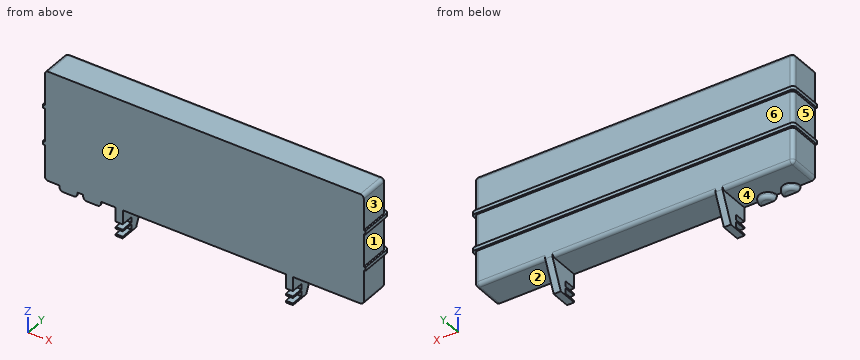
Autodesk Fusion 360 part; units mm, degrees
sketch "Sketch1" plane through (0, 0, 0) normal (0, 1, 0) x (1, 0, 0)
  line L0 (0, 0) -> (90, 0)
  line L1 (90, 0) -> (90, 31)
  line L2 (90, 31) -> (0, 31)
  line L3 (0, 31) -> (0, 0)
  line L4 (-3, 20.67) -> (93, 20.67) construction
  line L5 (-3, 10.33) -> (93, 10.33) construction
  line L6 (0, 21.17) -> (90, 21.17)
  line L7 (0, 20.17) -> (90, 20.17)
  line L8 (0, 9.83) -> (90, 9.83)
  line L9 (0, 10.83) -> (90, 10.83)
  line L10 (90, 20.17) -> (90.5, 20.17)
  line L11 (90.5, 20.17) -> (90.5, 21.17)
  line L12 (90.5, 21.17) -> (90, 21.17)
  line L13 (90, 21.17) -> (90, 20.17)
  line L14 (90, 10.83) -> (90.5, 10.83)
  line L15 (90.5, 10.83) -> (90.5, 9.83)
  line L16 (90.5, 9.83) -> (90, 9.83)
  line L17 (90, 9.83) -> (90, 10.83)
  line L18 (0, 21.17) -> (-0.5, 21.17)
  line L19 (-0.5, 21.17) -> (-0.5, 20.17)
  line L20 (-0.5, 20.17) -> (0, 20.17)
  line L21 (0, 20.17) -> (0, 21.17)
  line L22 (0, 9.83) -> (-0.5, 9.83)
  line L23 (-0.5, 9.83) -> (-0.5, 10.83)
  line L24 (-0.5, 10.83) -> (0, 10.83)
  line L25 (0, 10.83) -> (0, 9.83)
  line L26 (70, 39) -> (68, 39)
  line L27 (68, 39) -> (68, 38.5)
  line L28 (68, 38.5) -> (70, 38.5)
  line L29 (70, 38.5) -> (70, 39)
  line L30 (68, 37) -> (70, 37)
  line L31 (70, 37) -> (70, 36.5)
  line L32 (70, 36.5) -> (68, 36.5)
  line L33 (68, 36.5) -> (68, 37)
  line L34 (20, 37) -> (22, 37)
  line L35 (22, 37) -> (22, 36.5)
  line L36 (22, 36.5) -> (20, 36.5)
  line L37 (20, 36.5) -> (20, 37)
  line L38 (20, 38.5) -> (22, 38.5)
  line L39 (22, 38.5) -> (22, 39)
  line L40 (22, 39) -> (20, 39)
  line L41 (20, 39) -> (20, 38.5)
  dimension "d1" = 90
  dimension "d2" = 31
  dimension "d3" = 10.33
  dimension "d4" = 10.33
  dimension "d5" = 0.5
  dimension "d6" = 0.5
  dimension "d7" = 0.5
  dimension "d8" = 0.5
  dimension "d9" = 0.5
  dimension "d10" = 0.5
  dimension "d11" = 0.5
  dimension "d12" = 0.5
  dimension "d84" = 0.5
  dimension "d86" = 8
  dimension "d88" = 2
  dimension "d89" = 0.5
  dimension "d90" = 0.5
  dimension "d91" = 20
  dimension "d92" = 20
  dimension "d93" = 20
  dimension "d94" = 0.5
  dimension "d95" = 8
  dimension "d96" = 6
  dimension "d97" = 6
extrude "Extrude1" add sketch "Sketch1" along normal blind 9 contours L1 L2 L3 L6 makes body 1
extrude "Extrude2" add sketch "Sketch1" along normal blind 9 separate body contours L1 L3 L7 L9 makes body 2
extrude "Extrude3" add sketch "Sketch1" along normal blind 9 separate body contours L0 L1 L3 L8 makes body 3
extrude "Extrude4" add sketch "Sketch1" along normal blind 9.5 contours L1 L3 L6 L7 L13 L21 bodies 1 2
extrude "Extrude5" add sketch "Sketch1" along normal blind 9.5 contours L1 L3 L8 L9 L17 L25 bodies 1 3
extrude "Extrude6" add sketch "Sketch1" along normal blind 9.5 contours L1 L10 L11 L12 L13 bodies 1
extrude "Extrude7" add sketch "Sketch1" along normal blind 9.5 contours L1 L14 L15 L16 L17 bodies 1
extrude "Extrude8" add sketch "Sketch1" along normal blind 9.5 contours L3 L18 L19 L20 L21 bodies 1
extrude "Extrude9" add sketch "Sketch1" along normal blind 9.5 contours L3 L22 L23 L24 L25 bodies 1
sketch "Sketch2" plane through (0, 0, 0) normal (1, 0, 0) x (0, 0, -1)
  line L0 (39, 0) -> (31, 0)
  line L1 (31, 0) -> (31, 5.5)
  line L2 (31, 5.5) -> (39, 5.5)
  line L3 (39, 5.5) -> (39, 0)
  line L4 (31, 9) -> (39, 5.5)
  line L5 (31, 9) -> (31, 5.5)
  line L6 (39, 0) -> (35, 0)
  line L7 (35, 0) -> (35, 3.5)
  line L8 (35, 3.5) -> (39, 3.5)
  line L9 (39, 3.5) -> (39, 0)
  point P0 (31, 0)
  dimension "d33" = 8
  dimension "d34" = 8
  dimension "d35" = 5.5
  dimension "d36" = 3.5
  dimension "d37" = 4
extrude "Extrude10" add sketch "Sketch2" along normal blind 2 from surface at 68 contours L0 L1 L2 L3 L7 L8 | L2 L4 L5 bodies 1
extrude "Extrude11" add sketch "Sketch2" along normal blind 2 from surface at 20 contours L0 L1 L2 L3 L7 L8 | L2 L4 L5 bodies 1
fillet "Fillet1" radius 1 1 edges at (90, 9, -4.915) on bodies 1
fillet "Fillet2" radius 1 1 edges at (90, 9, -15.5) on bodies 1
fillet "Fillet3" radius 1 1 edges at (90, 9, -26.085) on bodies 1
fillet "Fillet4" radius 1 3 edges at (90, 4, -31) (89.7071, 8.7071, -31) (79.5, 9, -31) on bodies 1
fillet "Fillet5" radius 1 3 edges at (90, 4, 0) (89.7071, 8.7071, 0) (44.5, 9, 0) on bodies 1
fillet "Fillet6" radius 1 3 edges at (0, 4, 0) (0, 8.7071, -0.2929) (0, 9, -5.415) on bodies 1
fillet "Fillet7" radius 1 1 edges at (0, 9, -15.5) on bodies 1
fillet "Fillet8" radius 1 1 edges at (0, 9, -26.085) on bodies 1
fillet "Fillet9" radius 1 3 edges at (0, 4, -31) (0.2929, 8.7071, -31) (10.5, 9, -31) on bodies 1
fillet "Fillet10" radius 1 1 edges at (45, 9, -31) on bodies 1
sketch "Sketch3" plane through (0, 0, -31) normal (0, 0, -1) x (-1, 0, 0)
  line L0 (-1, 8) -> (-20, 8)
  line L1 (-20, 8) -> (-20, 0)
  line L2 (-20, 0) -> (-1, 0)
  line L3 (-1, 0) -> (-1, 8)
  line L4 (-6.666, -3) -> (-6.666, 13) construction
  line L5 (-13.333, -2) -> (-13.333, 13) construction
  circle A0 centre (-6.666, 0) radius 2.5
  circle A1 centre (-13.333, 0) radius 2.5
  dimension "d64" = 6.667
  dimension "d65" = 6.667
  dimension "d66" = 5
  dimension "d67" = 5
extrude "Extrude12" add sketch "Sketch3" along normal blind 1.5 contours L2 A0 picked at (-6.0551, 0.5668) bodies 1
extrude "Extrude13" add sketch "Sketch3" along normal blind 1.5 contours L2 A1 picked at (-12.6445, 0.4694) bodies 1
fillet "Fillet11" radius 1 1 edges at (6.666, 2.5, -32.5) on bodies 1
fillet "Fillet12" radius 1 1 edges at (13.333, 2.5, -32.5) on bodies 1
fillet "Fillet13" radius 1 1 edges at (90.5, 9.5, -20.67) on bodies 1
fillet "Fillet14" radius 1 1 edges at (90.5, 9.5, -10.33) on bodies 1
fillet "Fillet15" radius 1 1 edges at (-0.5, 9.5, -20.67) on bodies 1
fillet "Fillet16" radius 1 1 edges at (-0.5, 9.5, -10.33) on bodies 1
extrude "Extrude14" add sketch "Sketch1" along normal blind 3.5 contours L26 L27 L28 L29 | L30 L31 L32 L33 bodies 1
extrude "Extrude15" add sketch "Sketch1" along normal blind 3.5 contours L34 L35 L36 L37 | L38 L39 L40 L41 bodies 1
Read the model definition and answer for the solid it produces. Units are mm, in the model's axes. Face numbers are marked on the shaded views. A direction names the side the tool comes from. Coordinates: 2 decimals unless noted, no trailing zeros. Write each loop counter-clockwise with the first axis right and the second up, starting at its lowest first coordinate (ties: lowest second). Pieces come first, ordered by that corner, then holes. Notation, with made-up numbers: (49.5, 37.5) -> (63.5, 37.5) arc R22 cw to (63.5, 46.5) -> close; hole circle Ø2 at (77.5, 16.25). An arc over 180 degrees is marked (long way). Answer as a JSON object with one key per item and string values.
Q1. A tool of negligible diameter and unlimited length cuts with its end or side. For the marked faces 1, 2 and 3, from which of +Z, -Z, +X, -X, +Y, -Y can it reach the whole face along a straight path? Write none if from no direction.
The answers:
{"face 1": "+X, +Y, -Y", "face 2": "-Z, +X, +Y, -Y", "face 3": "+Z, +X, +Y, -Y"}
Q2. The part is cut by section B-B on x = 18. Give the vertices of the cut face in (y, z), then the cut area to 3 significant figures.
The answers:
{"outline": "(0, -31) -> (8, -31) arc R1 ccw to (9, -30) -> (9, -21.17) -> (9.5, -21.17) -> (9.5, -20.17) -> (9, -20.17) -> (9, -10.83) -> (9.5, -10.83) -> (9.5, -9.83) -> (9, -9.83) -> (9, -1) arc R1 ccw to (8, 0) -> (0, 0) -> close", "area": "280 mm2"}
Q3. Determine the mould class of the marked faces 4, 5, 6 and 7 for opening direction Z: pulls with the +Z half, pulls with the -Z half, needs draft (parallel to the pull), parting line crosses it, or undercut.
The answers:
{"face 4": "pulls with the -Z half", "face 5": "undercut", "face 6": "undercut", "face 7": "needs draft"}
Q4. Consider line 1 (Z direction, x = 36.5, y = 7); line 2 (X direction, y = 6.75, z = -25); line 3 (Y direction, x = 9, z = -23). Determine where each line is inside the solid, lowest interval first. Write a range as [from, to].
The answers:
{"line 1": "z = [-31, 0]", "line 2": "x = [0, 90]", "line 3": "y = [0, 9]"}
Q5. The part is cut by section C-C on z = -9. Give the vertices of the cut face in (x, y), then the cut area to 3 significant figures.
The answers:
{"outline": "(0, 0) -> (90, 0) -> (90, 8) arc R1 ccw to (89, 9) -> (1, 9) arc R1 ccw to (0, 8) -> close", "area": "810 mm2"}
Q6. Flat-ended cylindrical pins translate along their axes: pin 1 Ø1 at (x, y) = (20.5, 1.5) entering from +Z; pin 2 Ø2.5 at (y, z) = (3, -7.5) entering from -X; pin 3 Ø8 at (x, z) = (68.5, -31.5) entering from +Y; pin 4 Ø4.5 at (y, z) = (3, -33) entering from +X. Find the tip coordinate at first contact, or state that the pin passes through.
The answers:
{"pin 1": "stops at z = 0", "pin 2": "stops at x = 0", "pin 3": "stops at y = 9", "pin 4": "stops at x = 89.66"}
